Source: three-view drawing plus pictorial views. Frame: mm from the lowest corner of the part. A direction names the side the tool comes from. Coordinates: 2 decimals unless noted, no trailing zeros. Write each loop counter-clockwise with the first axis right and the second up, starting at its lowest first coordinate (ties: lowest second). Pieces come first, ordered by that corner, then holes. Notation, with made-up numbers: (19, 41) -> (76, 41) arc R22 cw to (76, 69) -> close; hole circle Ø8 at (28, 74). An arc over 180 degrees is marked (long way). Write item = value, one per line.
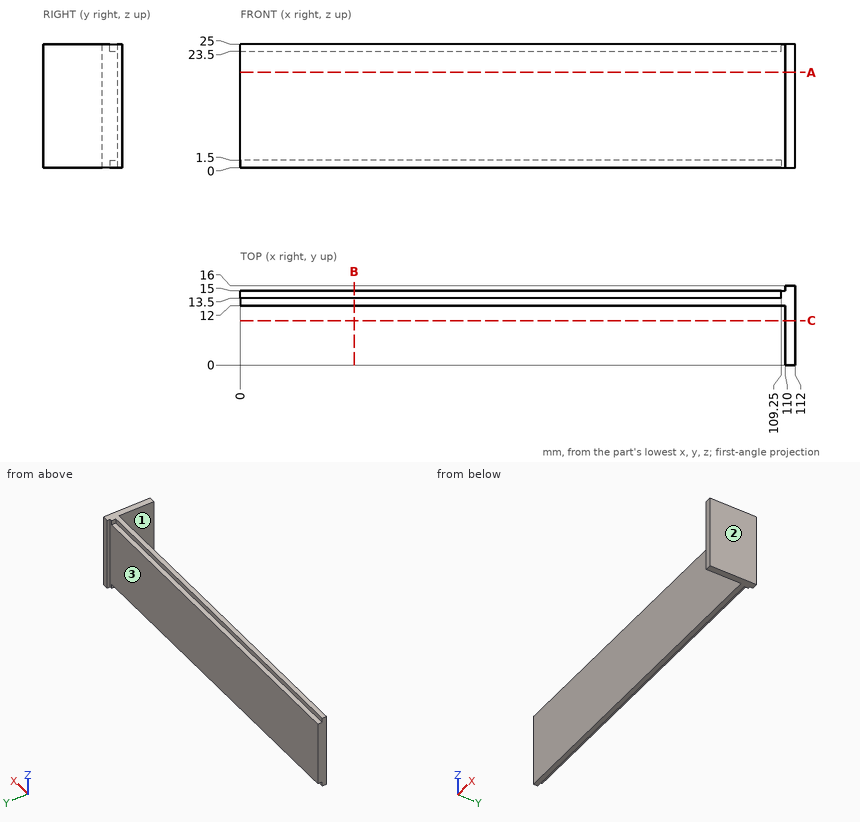
1) Cut plane C-C, the plane y = 9. Output: boundary loops of the cut face in (x, z), and give its area (3 significant figures).
Answer block:
outline = (110, 0) -> (112, 0) -> (112, 25) -> (110, 25) -> close
area = 50.0 mm2
2) Cut plane B-B, the plane x = 23. Output: boundary loops of the cut face in (y, z).
Answer block:
outline = (12, 0) -> (13.5, 0) -> (13.5, 1.5) -> (15, 1.5) -> (15, 23.5) -> (13.5, 23.5) -> (13.5, 25) -> (12, 25) -> close
3) Cut plane A-A, the plane z = 19.25. Output: boundary loops of the cut face in (x, y).
Answer block:
outline = (0, 12) -> (110, 12) -> (110, 0) -> (112, 0) -> (112, 16) -> (110, 16) -> (110, 15) -> (0, 15) -> close
4) Reachability of the marked faces 1, 2 and 3 from +Z, -Z, +X, -X, +Y, -Y: full face, straight path, thin tool, end or side. Return the list, or none.
Answer block:
face_1 = +Z, -Z, -X, -Y
face_2 = +Z, -Z, +X, +Y, -Y
face_3 = +Z, -Z, -X, +Y
5) First-contact query: pin 1 Ø5 at (y, z) = (10, 14) entering from -X; pin 2 Ø12.5 at (x, z) = (51, 12.5) entering from -Y; pin 3 Ø0.8 at (x, y) = (60, 14) entering from -Z; pin 4 Ø4 at (y, z) = (7, 21.5) entering from -X. Flat tips, straight axial feed; report the tip coordinate or a pass-through.
Answer block:
pin_1 = 0
pin_2 = 12
pin_3 = 1.5
pin_4 = 110
6) Material intervals for probe 1 along Y at (x, z) = (77.5, 19); probe 2 along X at (y, z) = (11.25, 9); probe 3 along Z at (x, y) = (77, 14.75), sorted ascending. Write a range as [from, to].
Answer block:
probe_1 = [12, 15]
probe_2 = [110, 112]
probe_3 = [1.5, 23.5]
